```python
from build123d import *

# Parameters (mm, degrees)
SKETCH1_R           = 6
BOSS_EXTRUDE2_DEPTH = 111
BOSS_EXTRUDE4_DEPTH = 0.5


with BuildPart() as part:
    # Sketch1 → Boss-Extrude2 (new body)
    with BuildSketch(Plane(origin=(0, 0, 0), x_dir=(1, 0, 0), z_dir=(0, 1, 0))):
        Circle(SKETCH1_R)
    boss_extrude2 = extrude(amount=BOSS_EXTRUDE2_DEPTH)

    # Sketch4 → Boss-Extrude4 (add, symmetric)
    with BuildSketch(Plane(origin=(0, 0, 0), x_dir=(-0.707106781, 0, -0.707106781), z_dir=(0.707106781, 0, -0.707106781))):
        with BuildLine():
            Line((5, -5), (5, 0))
            Line((5, 0), (6, 0))
            Line((6, 0), (6, -5))
            add(Edge.make_bspline(
                [(-6, -5), (-6, -10), (0, -10), (6, -10), (6, -5)],
                knots=[3.141592654, 3.141592654, 3.141592654, 4.71238898, 4.71238898, 6.283185307, 6.283185307, 6.283185307], degree=2, weights=[1, 0.707106781, 1, 0.707106781, 1]))
            Line((-6, -5), (-6, 0))
            Line((-6, 0), (-5, 0))
            Line((-5, 0), (-5, -5))
            add(Edge.make_bspline(
                [(-5, -5), (-5, -9), (0, -9), (5, -9), (5, -5)],
                knots=[3.141592654, 3.141592654, 3.141592654, 4.71238898, 4.71238898, 6.283185307, 6.283185307, 6.283185307], degree=2, weights=[1, 0.707106781, 1, 0.707106781, 1]))
        make_face()
    boss_extrude4 = extrude(amount=BOSS_EXTRUDE4_DEPTH, both=True)

    # Mirror1: Boss-Extrude2, Boss-Extrude4 across plane
    add(boss_extrude2.mirror(Plane.ZX.offset(111)))
    add(boss_extrude4.mirror(Plane.ZX.offset(111)))


solid = part.part
```
Source: CAD feature listing. Evaluate the final solid. Frame: model axes, mm. A direction names the side the tool comes from. Round coordinates to 2 decimals unless told otherwise and drop trailing zeros. Loops run counter-clockwise (first coordinate to the right, second up) from the corner with the lowest first, then second, coordinate; pieces in that order, holes last.
1. Section query A-A on y = 200. Output: boundary loops of the cut face in (x, z), and give its area (3 significant figures).
2. Ray query, L1, parallel to Z at x = 0.5, y = 14.5; L2, parallel to Y at x = -5, z = 2.5; L3, parallel to X at y = 144.5, z = 0.75. Return the intervals inside material, ascending.
3. Access query for faces 1 (the flat face through (0.569, -9.051, 1.277)), 2 (the flat face through (1.277, 231.051, 0.569)), 3 (the flat face through (0.569, 231.051, 1.277)), 4 (the flat face through (1.277, -9.051, 0.569)). Directions: +Z, -Z, +X, -X, +Y, -Y. A direction counts if a zero-diameter tool reaches every point of the face in a straight line with its end or side. Return the directions, or none.
4. Contact query for flat-ended pins moving along their axis: pin 1 (1.5 mm diameter, centred on x = 3, y = 90.5, fed in from -Z); pin 2 (2 mm diameter, centred on x = -1, z = -2, fed in from +Y); pin 3 (1 mm diameter, centred on x = 4, z = -4, fed in from -Y). Output: stop coordinate, or through.
Answers below:
1. outline: circle Ø12 at (0, 0)
1. area: 113 mm2
2. L1: z = -5.98 to 5.98
2. L2: y = 0 to 222
2. L3: x = -5.95 to 5.95
3. face 1: +Z, -X, -Y
3. face 2: -Z, +X, +Y
3. face 3: +Z, -X, +Y
3. face 4: -Z, +X, -Y
4. pin 1: stops at z = -5.56
4. pin 2: stops at y = 231.91
4. pin 3: stops at y = 0
